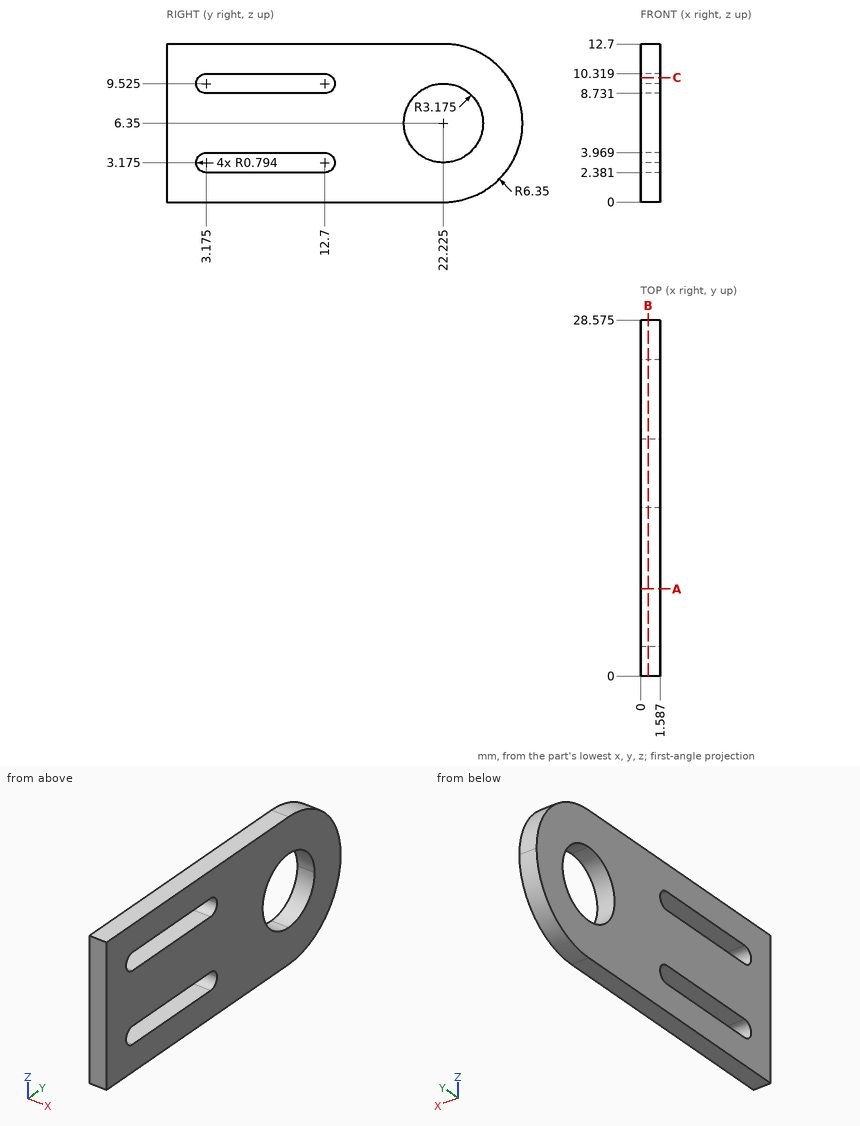
Can you work these out from the drawing? Everything is in mm from the part's minimum corner. Round coordinates to 2 decimals unless told otherwise and drop trailing zeros. Loops run counter-clockwise (first coordinate to the right, second up) from the corner with the lowest first, then second, coordinate; pieces in that order, holes last.
1. If we section it at B-B on x = 0.6: Count the separate pieces of the cut face and the enclosed holes in it, plus the area to 3 significant figures.
Answer list:
separate pieces: 1
enclosed holes: 3
area: 280 mm2
2. For P1, Ø1, axis at y = 20.5, z = 5, coming from the +X side, with a flat end and sliding along its axis, tell me the tip position at first contact or that it passes through.
Answer list:
P1: passes through
3. If we section it at A-A on y = 7: Write out the boundary of the cut face in (x, z).
Answer list:
outline: (0, 0) - (1.59, 0) - (1.59, 2.38) - (0, 2.38) - close; (0, 3.97) - (1.59, 3.97) - (1.59, 8.73) - (0, 8.73) - close; (0, 10.32) - (1.59, 10.32) - (1.59, 12.7) - (0, 12.7) - close
4. If I drill on line 1 along Z through (x, y) = (1.2, 12.5); line 2 along Y through (x, z) = (1.3, 6.5); line 3 along Z through (x, y) = (1.4, 2.75) (1 decimal), over which ranges is the centre line in solid material (lowest first)?
Answer list:
line 1: z = 0 to 2.38, 3.97 to 8.73, 10.32 to 12.7
line 2: y = 0 to 19.05, 25.4 to 28.57
line 3: z = 0 to 2.5, 3.8 to 8.9, 10.2 to 12.7
5. If we section it at C-C on z = 10: Write out the boundary of the cut face in (x, y) (1 decimal), plus the area to 3 significant figures.
Answer list:
outline: (0, 0) - (1.6, 0) - (1.6, 2.5) - (0, 2.5) - close; (0, 13.3) - (1.6, 13.3) - (1.6, 27.4) - (0, 27.4) - close
area: 26.4 mm2
